Model file for the job. Use its own axes, mm. A direction names the side the tool comes from. Give positions to 0.01 mm unless a question says otherwise; leave off trailing zeros. Loops run counter-clockwise (first coordinate to the right, second up) from the corner with the lowest first, then second, coordinate; pieces in that order, holes last. Notation, with made-up numbers: M -4.75,83.25 L 5.25,83.25 A32 cw 5.25,113.25 Z; hole C 30.5,6 d8. An arc over 180 degrees is marked long. Answer in a Markdown table with one row per item.
```python
from build123d import *

# Parameters (mm, degrees)
SKETCH1_W                = 368.3
SKETCH1_H                = 31.75
BOSS_EXTRUDE1_DEPTH      = 368.3
SHELL1_T                 = -31.75
BOSS_EXTRUDE2_DEPTH      = 418.3
BOSS_EXTRUDE2_DEPTH_BACK = 50


with BuildPart() as part:
    # Sketch1 → Boss-Extrude1 (new body)
    with BuildSketch(Plane.XY):
        with Locations((184.15, 15.875)):
            Rectangle(SKETCH1_W, SKETCH1_H)
    extrude(amount=BOSS_EXTRUDE1_DEPTH)

    # Shell1
    shell1_openings = [part.faces().sort_by_distance(p)[0] for p in [
        (184.15, 31.75, 184.15),
        (184.15, 0, 184.15),
    ]]
    offset(amount=SHELL1_T, openings=shell1_openings, kind=Kind.INTERSECTION)

    # Sketch2 → Boss-Extrude2 (add, two sides: drawn at the far end of the back side and taken through both)
    with BuildSketch(Plane.XY.offset(-BOSS_EXTRUDE2_DEPTH_BACK)):
        Polygon((368.3, 31.75), (388.3, 31.75), (418.3, 107.95), (37.3, 107.95), (-52.7, 793.75), (-120, 793.75), (-20, 31.75), (0, 31.75), align=None)
    extrude(amount=BOSS_EXTRUDE2_DEPTH + BOSS_EXTRUDE2_DEPTH_BACK)


solid = part.part
```
Q1. Probe probe 1 along Y at (x, z) = (213, 266.5); probe 2 along Y at (x, z) = (248, 367); probe 3 along X at (y, z) = (514, 43). List the from-to ranges inside material, lowest first.
Reported:
| item | result |
|---|---|
| probe 1 | 31.75 to 107.95 |
| probe 2 | 0 to 107.95 |
| probe 3 | -83.29 to -15.99 |
Q2. Saw through at C-C (x = 356.5). Give the cut face in (y, z), and give its area (3 significant figures).
Reported:
| item | result |
|---|---|
| outline | M 0,0 L 31.75,0 L 31.75,-50 L 107.95,-50 L 107.95,418.3 L 31.75,418.3 L 31.75,368.3 L 0,368.3 Z |
| area | 47,400 mm² |
Q3. 3-axis set-ups, long thin cutter, end or side, ignore diameter. For faces 1 (the face through (182, 16, 0)), 2 (the face through (0, 16, 182)), 3 (the face through (336.55, 16, 182)), 4 (the face through (230, 107.95, 181)): which of +Z, -Z, +X, -X, +Y, -Y reach the whole face in a straight line?
Reported:
| item | result |
|---|---|
| face 1 | -Z, +X, -X, -Y |
| face 2 | +Z, -Z, -X, -Y |
| face 3 | -Y |
| face 4 | +Z, -Z, +X, +Y |
Q4. Drop flat-ended pins along their axis: pin 1 (1.5 mm diameter, centred on y = 347.5, z = 336.5, fed in from -X); pin 2 (9.5 mm diameter, centred on x = 234, y = 17, fed in from +Z); pin 3 (2 mm diameter, centred on x = 359, z = 98, fed in from +Y). Give the stop position or say it passes through.
Reported:
| item | result |
|---|---|
| pin 1 | x = -61.54 |
| pin 2 | z = 368.3 |
| pin 3 | y = 107.95 |
Q5. Saw through at D-D (z = 352). Give the cut face in (x, y), and give its area (3 significant figures).
Reported:
| item | result |
|---|---|
| outline | M -120,793.75 L -20,31.75 L 0,31.75 L 0,0 L 368.3,0 L 368.3,31.75 L 388.3,31.75 L 418.3,107.95 L 37.3,107.95 L -52.7,793.75 Z |
| area | 90,500 mm² |
Q6. Saw through at A-A (x = 184). Give the cut face in (y, z), and give its area (3 significant figures).
Reported:
| item | result |
|---|---|
| outline | M 0,0 L 31.75,0 L 31.75,-50 L 107.95,-50 L 107.95,418.3 L 31.75,418.3 L 31.75,368.3 L 0,368.3 L 0,336.55 L 31.75,336.55 L 31.75,31.75 L 0,31.75 Z |
| area | 37,700 mm² |
Q7. Saw through at B-B (z = 102.5). Give the cut face in (x, y).
Reported:
| item | result |
|---|---|
| outline | M -120,793.75 L -20,31.75 L 0,31.75 L 0,0 L 31.75,0 L 31.75,31.75 L 336.55,31.75 L 336.55,0 L 368.3,0 L 368.3,31.75 L 388.3,31.75 L 418.3,107.95 L 37.3,107.95 L -52.7,793.75 Z |
Q8. Mould opens along Z. For faces 5 (the face through (182, 31.75, 182)), 6 (the face through (368.3, 16, 182)), 7 (the face through (8, 273, -50)) say: released by +Z, released by -Z, zero draft, split by the parting line, or undercut.
Reported:
| item | result |
|---|---|
| face 5 | undercut |
| face 6 | zero draft |
| face 7 | released by -Z |
